```python
from build123d import *

# Parameters (mm, degrees)
SKETCH_1_W           = 67.5
SKETCH_1_H           = 62.5
EXTRUDE_1_DEPTH      = 1.6
SKETCH_2_R           = 1.65
CUT_EXTRUDE_1_DEPTH  = 10
CHAMFER_1_SIZE       = 3
SKETCH_3_R           = 1.65
EXTRUDE_2_DEPTH      = 4
SKETCH_4_R           = 4
CUT_EXTRUDE_2_DEPTH  = 0.8
SKETCH_5_R           = 4.5
EXTRUDE_3_DEPTH      = 6
EXTRUDE_4_DEPTH      = 8
SKETCH_7_W           = 10
SKETCH_7_H           = 1
CUT_EXTRUDE_3_DEPTH  = 5
EXTRUDE_5_DEPTH      = 2
CUT_EXTRUDE_4_DEPTH  = 8
FILLET_2_R           = 2
EXTRUDE_7_DEPTH      = 2
EXTRUDE_7_DEPTH_BACK = 2
SKETCH_12_R          = 4.5
SKETCH_12_R_2        = 1.65


with BuildPart() as part:
    # 草图1 → 凸台-拉伸1 (new body)
    with BuildSketch(Plane.XY):
        Rectangle(SKETCH_1_W, SKETCH_1_H)
    extrude(amount=EXTRUDE_1_DEPTH)

    # 草图2 → 切除-拉伸1 (cut)
    with BuildSketch(Plane.XY.offset(1.6)):
        with Locations((-22.5, 20)):
            Circle(SKETCH_2_R)
        with Locations((22.5, 20)):
            Circle(SKETCH_2_R)
        with Locations((22.5, -20)):
            Circle(SKETCH_2_R)
        with Locations((-22.5, -20)):
            Circle(SKETCH_2_R)
        Polygon((-30.75, 11.25), (-30.75, -11.25), (-33.75, -14.25), (-33.75, 14.25), align=None)
        Polygon((30.75, 11.25), (30.75, -11.25), (33.75, -14.25), (33.75, 14.25), align=None)
    extrude(amount=-CUT_EXTRUDE_1_DEPTH, mode=Mode.SUBTRACT)

    # 倒角1
    chamfer_1_edges = [part.edges().sort_by_distance(p)[0] for p in [
        (33.75, -31.25, 0.8),
        (-33.75, -31.25, 0.8),
        (-33.75, 31.25, 0.8),
        (33.75, 31.25, 0.8),
    ]]
    chamfer(chamfer_1_edges, length=CHAMFER_1_SIZE)

    # 草图3 → 凸台-拉伸2 (add)
    # profile 1 of 4: a face of its own
    with BuildSketch(Plane(origin=(0, 0, 0), x_dir=(-1, 0, 0), z_dir=(0, 0, -1))):
        Polygon((-19.901923789, 20), (-21.200961894, 22.25), (-23.799038106, 22.25), (-25.098076211, 20), (-23.799038106, 17.75), (-21.200961894, 17.75), align=None)
        with Locations(Location((-22.5, 20, 0), (0, 0, 180))):
            Circle(SKETCH_3_R, mode=Mode.SUBTRACT)
    # profile 2 of 4: a face of its own
    with BuildSketch(Plane(origin=(0, 0, 0), x_dir=(-1, 0, 0), z_dir=(0, 0, -1))):
        Polygon((25.098076211, 20), (23.799038106, 22.25), (21.200961894, 22.25), (19.901923789, 20), (21.200961894, 17.75), (23.799038106, 17.75), align=None)
        with Locations(Location((22.5, 20, 0), (0, 0, 180))):
            Circle(SKETCH_3_R, mode=Mode.SUBTRACT)
    # profile 3 of 4: a face of its own
    with BuildSketch(Plane(origin=(0, 0, 0), x_dir=(-1, 0, 0), z_dir=(0, 0, -1))):
        Polygon((25.098076211, -20), (23.799038106, -17.75), (21.200961894, -17.75), (19.901923789, -20), (21.200961894, -22.25), (23.799038106, -22.25), align=None)
        with Locations(Location((22.5, -20, 0), (0, 0, 180))):
            Circle(SKETCH_3_R, mode=Mode.SUBTRACT)
    # profile 4 of 4: a face of its own
    with BuildSketch(Plane(origin=(0, 0, 0), x_dir=(-1, 0, 0), z_dir=(0, 0, -1))):
        Polygon((-19.901923789, -20), (-21.200961894, -17.75), (-23.799038106, -17.75), (-25.098076211, -20), (-23.799038106, -22.25), (-21.200961894, -22.25), align=None)
        with Locations(Location((-22.5, -20, 0), (0, 0, 180))):
            Circle(SKETCH_3_R, mode=Mode.SUBTRACT)
    extrude(amount=EXTRUDE_2_DEPTH)

    # 草图4 → 切除-拉伸2 (cut)
    with BuildSketch(Plane.XY.offset(1.6)):
        with Locations((-22.5, 20)):
            Circle(SKETCH_4_R)
        with Locations((22.5, 20)):
            Circle(SKETCH_4_R)
        with Locations((22.5, -20)):
            Circle(SKETCH_4_R)
        with Locations((-22.5, -20)):
            Circle(SKETCH_4_R)
    extrude(amount=-CUT_EXTRUDE_2_DEPTH, mode=Mode.SUBTRACT)

    # 草图5 → 凸台-拉伸3 (add)
    # profile 1 of 4: a face of its own
    with BuildSketch(Plane(origin=(0, 0, 0), x_dir=(-1, 0, 0), z_dir=(0, 0, -1))):
        with Locations(Location((-22.5, 20, 0), (0, 0, 180))):
            Circle(SKETCH_5_R)
        Polygon((-21.200961894, 17.75), (-19.901923789, 20), (-21.200961894, 22.25), (-23.799038106, 22.25), (-25.098076211, 20), (-23.799038106, 17.75), align=None, mode=Mode.SUBTRACT)
    # profile 2 of 4: a face of its own
    with BuildSketch(Plane(origin=(0, 0, 0), x_dir=(-1, 0, 0), z_dir=(0, 0, -1))):
        with Locations(Location((22.5, 20, 0), (0, 0, 180))):
            Circle(SKETCH_5_R)
        Polygon((23.799038106, 17.75), (25.098076211, 20), (23.799038106, 22.25), (21.200961894, 22.25), (19.901923789, 20), (21.200961894, 17.75), align=None, mode=Mode.SUBTRACT)
    # profile 3 of 4: a face of its own
    with BuildSketch(Plane(origin=(0, 0, 0), x_dir=(-1, 0, 0), z_dir=(0, 0, -1))):
        with Locations(Location((22.5, -20, 0), (0, 0, 180))):
            Circle(SKETCH_5_R)
        Polygon((23.799038106, -22.25), (25.098076211, -20), (23.799038106, -17.75), (21.200961894, -17.75), (19.901923789, -20), (21.200961894, -22.25), align=None, mode=Mode.SUBTRACT)
    # profile 4 of 4: a face of its own
    with BuildSketch(Plane(origin=(0, 0, 0), x_dir=(-1, 0, 0), z_dir=(0, 0, -1))):
        with Locations(Location((-22.5, -20, 0), (0, 0, 180))):
            Circle(SKETCH_5_R)
        Polygon((-21.200961894, -22.25), (-19.901923789, -20), (-21.200961894, -17.75), (-23.799038106, -17.75), (-25.098076211, -20), (-23.799038106, -22.25), align=None, mode=Mode.SUBTRACT)
    extrude(amount=EXTRUDE_3_DEPTH)

    # 草图6 → 凸台-拉伸4 (add)
    with BuildSketch(Plane(origin=(0, 0, 0), x_dir=(-1, 0, 0), z_dir=(0, 0, -1))):
        Polygon((-30.75, -31.25), (30.75, -31.25), (33.75, -28.25), (33.75, -14.25), (30.75, -11.25), (30.75, 11.25), (33.75, 14.25), (33.75, 28.25), (30.75, 31.25), (-30.75, 31.25), (-33.75, 28.25), (-33.75, 14.25), (-30.75, 11.25), (-30.75, -11.25), (-33.75, -14.25), (-33.75, -28.25), align=None)
        Polygon((-30.335786438, -30.25), (30.335786438, -30.25), (32.75, -27.835786438), (32.75, -14.664213562), (29.75, -11.664213562), (29.75, 11.664213562), (32.75, 14.664213562), (32.75, 27.835786438), (30.335786438, 30.25), (-30.335786438, 30.25), (-32.75, 27.835786438), (-32.75, 14.664213562), (-29.75, 11.664213562), (-29.75, -11.664213562), (-32.75, -14.664213562), (-32.75, -27.835786438), align=None, mode=Mode.SUBTRACT)
    extrude(amount=EXTRUDE_4_DEPTH)

    # 草图7 → 切除-拉伸3 (cut)
    with BuildSketch(Plane(origin=(0, 0, -8), x_dir=(-1, 0, 0), z_dir=(0, 0, -1))):
        with Locations((0, -30.75)):
            Rectangle(SKETCH_7_W, SKETCH_7_H)
    extrude(amount=-CUT_EXTRUDE_3_DEPTH, mode=Mode.SUBTRACT)

    # 草图8 → 凸台-拉伸5 (add)
    with BuildSketch(Plane(origin=(0, 0, 0), x_dir=(-1, 0, 0), z_dir=(0, 0, -1))):
        with BuildLine():
            Line((-1.5, -11.14955156), (-1.5, -12.157816416))
            ThreePointArc((-1.5, -12.157816416), (0, 12.25), (1.5, -12.157816416))
            Line((1.5, -12.157816416), (1.5, -11.14955156))
            ThreePointArc((1.5, -11.14955156), (0, 11.25), (-1.5, -11.14955156))
        make_face()
    extrude(amount=EXTRUDE_5_DEPTH)

    # 草图9 → 切除-拉伸4 (cut)
    with BuildSketch(Plane(origin=(0, 0, -8), x_dir=(-1, 0, 0), z_dir=(0, 0, -1))):
        Polygon((29.75, 11.664213562), (32.335786438, 14.25), (33.042893219, 13.542893219), (30.75, 11.25), (30.75, -11.25), (33.042893219, -13.542893219), (32.335786438, -14.25), (29.75, -11.664213562), align=None)
        Polygon((-33.042893219, 13.542893219), (-32.335786438, 14.25), (-29.75, 11.664213562), (-29.75, -11.664213562), (-32.335786438, -14.25), (-33.042893219, -13.542893219), (-30.75, -11.25), (-30.75, 11.25), align=None)
    extrude(amount=-CUT_EXTRUDE_4_DEPTH, mode=Mode.SUBTRACT)

    # 圆角2
    fillet_2_edges = [part.edges().sort_by_distance(p)[0] for p in [
        (5, -30.75, -3),
        (-5, -30.75, -3),
    ]]
    fillet(fillet_2_edges, radius=FILLET_2_R)

    # 草图12 → 凸台-拉伸7 (add, two sides: drawn at the far end of the back side and taken through both)
    # profile 1 of 4: a face of its own
    with BuildSketch(Plane(origin=(0, 0, -6), x_dir=(-1, 0, 0), z_dir=(0, 0, -1)).offset(-EXTRUDE_7_DEPTH_BACK)):
        with Locations(Location((-22.5, 20, 0), (0, 0, 180))):
            Circle(SKETCH_12_R)
        with Locations(Location((-22.5, 20, 0), (0, 0, 180))):
            Circle(SKETCH_12_R_2, mode=Mode.SUBTRACT)
    # profile 2 of 4: a face of its own
    with BuildSketch(Plane(origin=(0, 0, -6), x_dir=(-1, 0, 0), z_dir=(0, 0, -1)).offset(-EXTRUDE_7_DEPTH_BACK)):
        with Locations(Location((22.5, 20, 0), (0, 0, 180))):
            Circle(SKETCH_12_R)
        with Locations(Location((22.5, 20, 0), (0, 0, 180))):
            Circle(SKETCH_12_R_2, mode=Mode.SUBTRACT)
    # profile 3 of 4: a face of its own
    with BuildSketch(Plane(origin=(0, 0, -6), x_dir=(-1, 0, 0), z_dir=(0, 0, -1)).offset(-EXTRUDE_7_DEPTH_BACK)):
        with Locations(Location((-22.5, -20, 0), (0, 0, 180))):
            Circle(SKETCH_12_R)
        with Locations(Location((-22.5, -20, 0), (0, 0, 180))):
            Circle(SKETCH_12_R_2, mode=Mode.SUBTRACT)
    # profile 4 of 4: a face of its own
    with BuildSketch(Plane(origin=(0, 0, -6), x_dir=(-1, 0, 0), z_dir=(0, 0, -1)).offset(-EXTRUDE_7_DEPTH_BACK)):
        with Locations(Location((22.5, -20, 0), (0, 0, 180))):
            Circle(SKETCH_12_R)
        with Locations(Location((22.5, -20, 0), (0, 0, 180))):
            Circle(SKETCH_12_R_2, mode=Mode.SUBTRACT)
    extrude(amount=EXTRUDE_7_DEPTH + EXTRUDE_7_DEPTH_BACK)


solid = part.part
```
Check sheet for the modelled part. Datum: model origin and axes. Units: mm. A direction names the side the tool comes from. Round coordinates to 2 decimals unless told otherwise and drop trailing zeros. Loops run counter-clockwise (first coordinate to the right, second up) from the corner with the lowest first, then second, coordinate; pieces in that order, holes last. Notation, with made-up numbers: (24.25, 44.25) -> (37.25, 44.25) arc R20 cw to (37.25, 73.25) -> close; hole circle Ø10 at (51.5, -17). An arc over 180 degrees is marked (long way). Answer in a Markdown table with one row per item.
Q1. Go/stop test with flat-tipped pins: P1, Ø0.8, axis at y = -11.5, z = -0.5, coming from the +X side; P2, Ø5, axis at x = -22.5, y = 20, coming from the +Z side. Record where each tip stops, or that it passes through.
Data:
| item | result |
|---|---|
| P1 | stops at x = 5.18 |
| P2 | stops at z = 0.8 |
Q2. Thickness scan on L1, parallel to Y at x = 22.5, z = 1.05; L2, parallel to Y at x = -22.5, z = -1.5; L3, parallel to Y at x = -6, z = -7. Record the ranges inside material, lowest first.
Data:
| item | result |
|---|---|
| L1 | y = -31.25 to -24, -16 to 16, 24 to 31.25 |
| L2 | y = -31.25 to -30.25, -24.5 to -21.65, -18.35 to -15.5, 15.5 to 18.35, 21.65 to 24.5, 30.25 to 31.25 |
| L3 | y = -31.25 to -30.25, 30.25 to 31.25 |
Q3. Sectioned sample at A-A on x = -22.5. Give the number of separate pieces and of enclosed holes in the cut face, then the cut area to 3 significant figures.
Data:
| item | result |
|---|---|
| separate pieces | 3 |
| enclosed holes | 0 |
| area | 189 mm^2 |
Q4. Release check for a two-part mould opening along Y. For faces 6 (the face through (33.3, 13.8, -1)), 7 (the face through (32, -30, -3)), 8 (the face through (0, 0, 1.6)) record: released by +Y, released by -Y, zero draft, split by the parting line, or undercut.
Data:
| item | result |
|---|---|
| face 6 | undercut |
| face 7 | released by -Y |
| face 8 | zero draft |
Q5. Sectioned sample at D-D on y = 0. Enter the section's corners in (x, z).
Data:
| item | result |
|---|---|
| outline | (-30.75, 0) -> (-12.25, 0) -> (-12.25, -2) -> (-11.25, -2) -> (-11.25, 0) -> (11.25, 0) -> (11.25, -2) -> (12.25, -2) -> (12.25, 0) -> (30.75, 0) -> (30.75, 1.6) -> (-30.75, 1.6) -> close |
Q6. Set-up check for faces 1 (the face through (-23, -18, -8)), 2 (the face through (-4.43, -30.74, -3.6)), 3 (the face through (0.52, 12.24, -0.99)), 4 (the face through (22, 18, 0.8)), 5 (the face through (0, 31.25, -3)): record each of +Z, -Z, +X, -X, +Y, -Y from which the full face is reachable in a straight line by a thin tool's end or side.
Data:
| item | result |
|---|---|
| face 1 | -Z, +X, -X, +Y, -Y |
| face 2 | -Z, -Y |
| face 3 | -Z |
| face 4 | +Z |
| face 5 | +Z, -Z, +X, -X, +Y |
